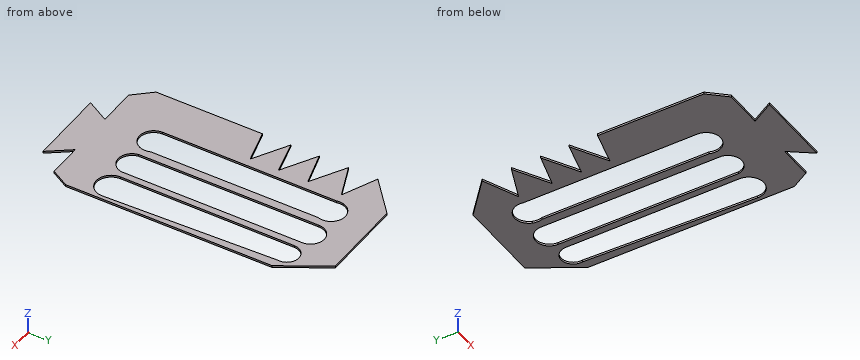
from build123d import *

# Parameters (mm, degrees)
F1_DEPTH = 1
F3_DEPTH = 1


with BuildPart() as f1:
    # F0 (on Top) → F1 (new body)
    with BuildSketch(Plane.XY):
        Polygon((12.651404, 85.822819), (-28.614573, 85.822819), (-45.86415, 70.602764), (-28.846802, 63.09859), (-45.86415, 56.122149), (-28.846802, 46.468406), (-45.86415, 41.641531), (-28.846802, 31.987788), (-45.86415, 27.599723), (-28.846802, 17.94598), (-45.86415, 13.503664), (-45.86415, -39.098875), (-38.06174, -47.875002), (-19.141939, -47.875002), (-25.34835, -58.81549), (12.651404, -58.81549), (4.502493, -47.875002), (21.428692, -47.875002), (26.407287, -39.098875), (26.407287, 63.09859), align=None)
    extrude(amount=F1_DEPTH)

    # F2 (on face) → F3 (cut)
    with BuildSketch(Plane.XY.offset(1)):
        with BuildLine():
            Line((-10.944886, 67.442728), (-10.944886, 62.627868))
            ThreePointArc((-10.944886, 62.627868), (-10.519625, 65.035298), (-10.944886, 67.442728))
        make_face()
        with BuildLine():
            Line((-10.944886, -20.112349), (-10.944886, 62.627868))
            Line((-10.944886, 62.627868), (-10.944886, 67.442728))
            ThreePointArc((-10.944886, 67.442728), (-17.969793, 72.049479), (-24.389813, 66.631471))
            Line((-24.389813, 66.631471), (-24.398557, 63.477087))
            Line((-24.398557, 63.477087), (-24.637369, -22.680704))
            ThreePointArc((-24.637369, -22.680704), (-16.239304, -29.669648), (-10.944886, -20.112349))
        make_face()
        with BuildLine():
            Line((-24.398557, 63.477087), (-24.389813, 66.631471))
            ThreePointArc((-24.389813, 66.631471), (-24.573473, 65.054776), (-24.398557, 63.477087))
        make_face()
        with BuildLine():
            Line((-6.775405, 65.73049), (-6.775405, -23.601575))
            ThreePointArc((-6.775405, -23.601575), (0, -29.413971), (6.775405, -23.601575))
            Line((6.775405, -23.601575), (6.775405, 65.73049))
            ThreePointArc((6.775405, 65.73049), (0, 72.505895), (-6.775405, 65.73049))
        make_face()
        with BuildLine():
            Line((10.182706, 63.992515), (9.907027, -22.191573))
            ThreePointArc((9.907027, -22.191573), (17.372692, -29.580637), (24.635973, -21.992544))
            Line((24.635973, -21.992544), (22.063504, 63.09859))
            ThreePointArc((22.063504, 63.09859), (16.604961, 69.949706), (10.182706, 63.992515))
        make_face()
    extrude(amount=-F3_DEPTH, mode=Mode.SUBTRACT)


solid = f1.part
Geometry check sheet. Reference: the model listing, model coordinates, mm. Coordinates: 2 decimals unless noted, no trailing zeros. Loops run counter-clockwise (first coordinate to the right, second up) from the corner with the lowest first, then second, coordinate; pieces in that order, holes last. Notation, with made-up numbers: (45.25, 81.25) - (59.25, 81.25) arc R17 cw to (59.25, 92.25) - close; hole circle Ø7 at (18, 42). An arc over 180 degrees is marked (long way). Use one line per item in the form item = value. Start each with the question number.
Item 1: Section check D-D, the plane y = -14. Enter the section's corners in (x, z).
Item 2: Section check C-C, the plane y = 12. Enter the section's corners in (x, z), and give its area (3 significant figures).
Item 3: Thickness scan on probe 1 along X at (y, z) = (-10.5, 0.55); probe 2 along X at (y, z) = (-25, 0.35); probe 3 along Y at (x, z) = (-17, 0.15). Record the ranges inside material, lowest first.
Item 4: Section check A-A, the plane x = 0. Enter the section's corners in (y, z).
Item 5: Section check B-B, the plane z = 0.15. Give the number of separate pieces and of enclosed holes in the cut face, and give its area (3 significant figures).
Computed:
q1.outline = (-45.86, 0) - (-24.61, 0) - (-24.61, 1) - (-45.86, 1) - close; (-10.94, 0) - (-6.78, 0) - (-6.78, 1) - (-10.94, 1) - close; (6.78, 0) - (9.93, 0) - (9.93, 1) - (6.78, 1) - close; (24.39, 0) - (26.41, 0) - (26.41, 1) - (24.39, 1) - close
q2.outline = (-45.86, 0) - (-24.54, 0) - (-24.54, 1) - (-45.86, 1) - close; (-10.94, 0) - (-6.78, 0) - (-6.78, 1) - (-10.94, 1) - close; (6.78, 0) - (10.02, 0) - (10.02, 1) - (6.78, 1) - close; (23.61, 0) - (26.41, 0) - (26.41, 1) - (23.61, 1) - close
q2.area = 31.5 mm2
q3.probe_1 = -45.86 to -24.6, -10.94 to -6.78, 6.78 to 9.94, 24.29 to 26.41
q3.probe_2 = -45.86 to -24.25, -10.84 to -6.41, 6.41 to 10.45, 24.09 to 26.41
q3.probe_3 = -58.82 to -29.77, 72.04 to 85.82
q4.outline = (-58.82, 0) - (-29.41, 0) - (-29.41, 1) - (-58.82, 1) - close; (72.51, 0) - (85.82, 0) - (85.82, 1) - (72.51, 1) - close
q5.separate_pieces = 1
q5.enclosed_holes = 3
q5.area = 5,190 mm2
